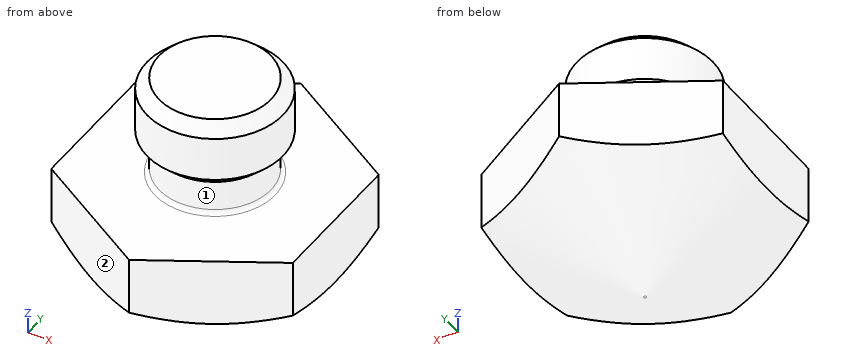
from build123d import *

# Parameters (mm, degrees)
SKETCH2_OUTSIDE_W  = 59.38
SKETCH2_OUTSIDE_H  = 59.38
CUT_EXTRUDE1_DEPTH = 13.7
FILLET1_R          = 0.381


with BuildPart() as part:
    # Sketch1 → Revolve1 (revolve)
    with BuildSketch(Plane(origin=(0, 0, 0), x_dir=(0, 0, -1), z_dir=(1, 0, 0)), mode=Mode.PRIVATE) as revolve1_sk:
        with BuildLine():
            Line((0, 22.065104351), (0, 5.1562))
            Line((0, 5.1562), (-3.175, 5.1562))
            Line((-3.175, 5.1562), (-4.2799, 6.2611))
            Line((-4.2799, 6.2611), (-8.4201, 6.2611))
            Line((-8.4201, 6.2611), (-9.525, 5.1562))
            Line((-9.525, 5.1562), (-9.525, 0))
            Line((-9.525, 0), (12.7, 0))
            ThreePointArc((12.7, 0), (12.69134516, 0.065740037), (12.665970453, 0.127))
            Line((12.665970453, 0.127), (0, 22.065104351))
        make_face()
    revolve(revolve1_sk.sketch.rotate(Axis((0, 0, 0), (0, 0, 1)), 90), axis=Axis((0, 0, 0), (0, 0, 1)))  # turned: the seam where the file's is

    # Sketch2 outside → Cut-Extrude1 (cut, through all)
    with BuildSketch(Plane.XY):
        Rectangle(SKETCH2_OUTSIDE_W, SKETCH2_OUTSIDE_H)
        Polygon((0, 12.831609733), (-11.1125, 6.415804866), (-11.1125, -6.415804866), (0, -12.831609733), (11.1125, -6.415804866), (11.1125, 6.415804866), align=None, mode=Mode.SUBTRACT)
    extrude(amount=-CUT_EXTRUDE1_DEPTH, mode=Mode.SUBTRACT)

    # Fillet1
    fillet1_edges = [part.edges().sort_by_distance(p)[0] for p in [
        (5.1562, 0, 0),
    ]]
    fillet(fillet1_edges, radius=FILLET1_R)


solid = part.part
Input: part model. Units: mm. Frame: model coordinates. Face numbers are marked on the shaded views. A direction names the side the tool comes from. Coordinates: 2 decimals unless noted, no trailing zeros. Loops run counter-clockwise (first coordinate to the right, second up) from the corner with the lowest first, then second, coordinate; pieces in that order, holes last.
(1) Material intervals for probe 1 along Z at (x, y) = (1.5, -8.5); probe 2 along Y at (x, z) = (-2.25, -3.5); probe 3 along Z at (x, y) = (-5, 5.5), sorted ascending.
(2) Section B-B on z = 2.75. Return the cut outline in (x, y).
(3) Section A-A on z = 8. Return the cut outline in (x, y).
(4) Set-up query: the marked faces 1 and 2. Return all of +Z, -Z, +X, -X, +Y, -Y with unobstructed straight access to the full face (end or side cutting, diameter ignored); none if empty.
(5) First-contact query: pin 1 Ø4 at (x, z) = (3, -1) entering from +Y; pin 2 Ø2 at (y, z) = (-3.5, 1.5) entering from -X; pin 3 Ø6 at (y, z) = (3, 1) entering from -X; pin 4 Ø6 at (x, z) = (-7.5, -3.5) entering from +Y. Flat tips, straight axial feed; report the tip coordinate or a pass-through.
Data:
1. probe 1: z = -7.76 to 0
1. probe 2: y = -11.53 to 11.53
1. probe 3: z = -8.45 to 0
2. outline: circle Ø10.31 at (0, 0)
3. outline: circle Ø12.52 at (0, 0)
4. face 1: none
4. face 2: +Z, -Z, -X, -Y
5. pin 1: stops at y = 12.25
5. pin 2: stops at x = -4.51
5. pin 3: stops at x = -11.11
5. pin 4: stops at y = 10.23
